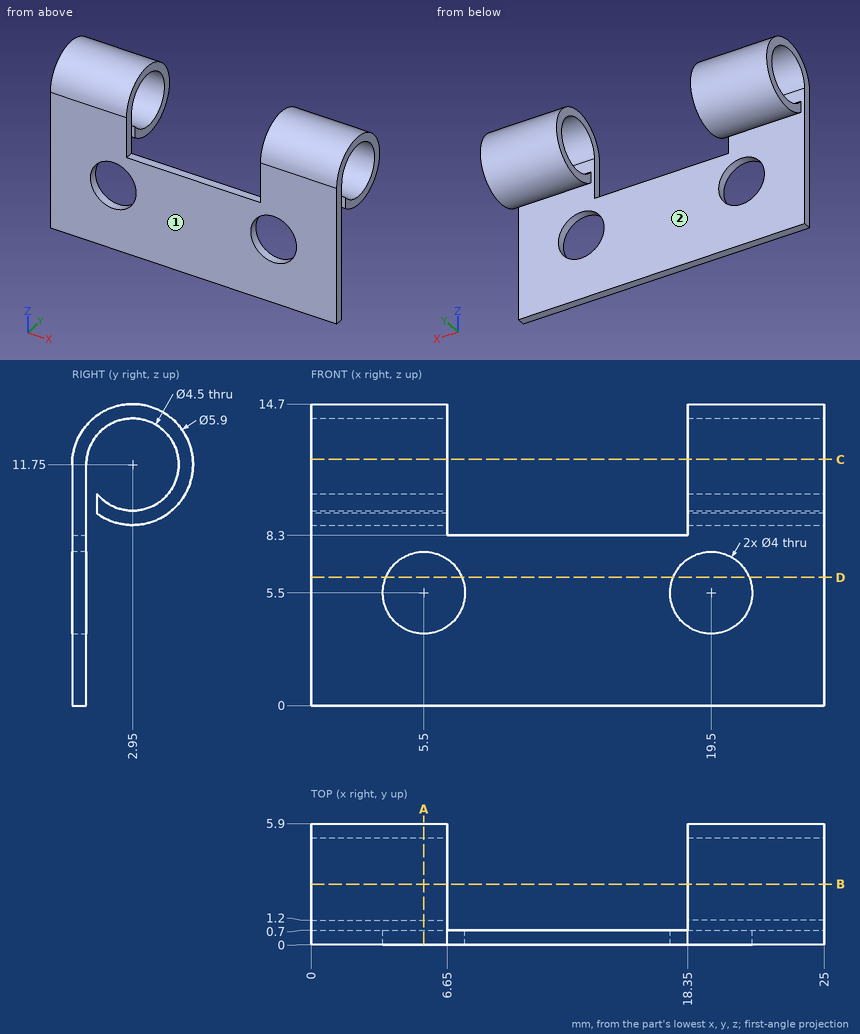
Can you work these out from the drawing? Everything is in mm from the part's minimum corner. Round coordinates to 2 decimals unless told otherwise and drop trailing zeros. Loops run counter-clockwise (first coordinate to the right, second up) from the corner with the lowest first, then second, coordinate; pieces in that order, holes last. Notation, with made-up numbers: (55.25, -9.75) - (94.25, -9.75) arc R20 ccw to (94.25, 26.25) - close; hole circle Ø10 at (-16.5, -24). An arc over 180 degrees is marked (long way). Answer in a Markdown table with one row per item. Add a question column.
Q1. I need wall thicknesses on L1, parallel to X at y = 0.4, z = 5.5; L2, parallel to Y at x = 23.75, z = 11.75; L3, parallel to Z at x = 2.5, y = 2.95. Which ranges of each line are inside material? Lowest first, please.
Q2. I want a section at C-C on z = 12. List the corners of the cut face in (x, y) for me.
Q3. I want a section at B-B on y = 2.95. List the corners of the cut face in (x, z) for me.
Q4. We'd pull the mould along Y, two halves only. Please class the marked faces 1 and 2: pulls with the +Y half, pulls with the -Y half, needs draft (parallel to the pull), parting line crosses it, or undercut.
Q5. For pin 1 Ø0.6 at (x, y) = (10.5, 0.5) entering from +Z; pin 2 Ø6 at (x, z) = (13, 4) entering from +Y, each with a flat end and sliding along its axis, tell me the tip position at first contact or that it passes through.
Q6. I want a section at A-A on x = 5.5. List the corners of the cut face in (y, z) for me, and give its area (3 significant figures).
Q7. I want a section at D-D on z = 6.25. List the corners of the cut face in (x, y) for me.
A:
| question | item | result |
|---|---|---|
| 1 | L1 | 0 to 3.5, 7.5 to 17.5, 21.5 to 25 |
| 1 | L2 | 0 to 0.7, 5.2 to 5.9 |
| 1 | L3 | 8.8 to 9.5, 14 to 14.7 |
| 2 | outline | (0, 0.01) - (6.65, 0.01) - (6.65, 0.71) - (0, 0.71) - close; (0, 5.19) - (6.65, 5.19) - (6.65, 5.89) - (0, 5.89) - close; (18.35, 0.01) - (25, 0.01) - (25, 0.71) - (18.35, 0.71) - close; (18.35, 5.19) - (25, 5.19) - (25, 5.89) - (18.35, 5.89) - close |
| 3 | outline | (0, 8.8) - (6.65, 8.8) - (6.65, 9.5) - (0, 9.5) - close; (0, 14) - (6.65, 14) - (6.65, 14.7) - (0, 14.7) - close; (18.35, 8.8) - (25, 8.8) - (25, 9.5) - (18.35, 9.5) - close; (18.35, 14) - (25, 14) - (25, 14.7) - (18.35, 14.7) - close |
| 4 | face 1 | pulls with the -Y half |
| 4 | face 2 | undercut |
| 5 | pin 1 | z = 8.3 |
| 5 | pin 2 | y = 0.7 |
| 6 | outline | (0, 0) - (0.7, 0) - (0.7, 3.5) - (0, 3.5) - close; (0, 7.5) - (0.7, 7.5) - (0.7, 11.75) arc R2.25 cw (long way) to (1.2, 10.34) - (1.2, 9.38) arc R2.95 ccw (long way) to (0, 11.75) - close |
| 6 | area | 15.3 mm^2 |
| 7 | outline | (0, 0) - (3.65, 0) - (3.65, 0.7) - (0, 0.7) - close; (7.35, 0) - (17.65, 0) - (17.65, 0.7) - (7.35, 0.7) - close; (21.35, 0) - (25, 0) - (25, 0.7) - (21.35, 0.7) - close |
